```python
from build123d import *

# Parameters (mm, degrees)
SKETCH1_W            = 20
SKETCH1_H            = 40
BOSS_EXTRUDE1_DEPTH  = 5
SKETCH2_W            = 20
SKETCH2_H            = 20
BOSS_EXTRUDE2_DEPTH  = 20
SKETCH3_W            = 6
SKETCH3_H            = 16
CUT_EXTRUDE1_DEPTH   = 20
M3_CLEARANCE_HOLE1_D = 3.4
SKETCH6_W            = 20
SKETCH6_H            = 5
BOSS_EXTRUDE3_DEPTH  = 60
SKETCH7_W            = 20
SKETCH7_H            = 5
BOSS_EXTRUDE4_DEPTH  = 20
SKETCH8_W            = 20
SKETCH8_H            = 20
BOSS_EXTRUDE5_DEPTH  = 20
SKETCH9_W            = 6
SKETCH9_H            = 16
CUT_EXTRUDE2_DEPTH   = 20
M3_CLEARANCE_HOLE2_D = 3.4


with BuildPart() as part:
    # Sketch1 → Boss-Extrude1 (new body)
    with BuildSketch(Plane(origin=(0, 0, 0), x_dir=(1, 0, 0), z_dir=(0, 1, 0))):
        Rectangle(SKETCH1_W, SKETCH1_H)
    extrude(amount=BOSS_EXTRUDE1_DEPTH)

    # Sketch2 → Boss-Extrude2 (add)
    with BuildSketch(Plane(origin=(0, 0, 0), x_dir=(-1, 0, 0), z_dir=(0, -1, 0))):
        with Locations((0, 10)):
            Rectangle(SKETCH2_W, SKETCH2_H)
    extrude(amount=BOSS_EXTRUDE2_DEPTH)

    # Sketch3 → Cut-Extrude1 (cut)
    with BuildSketch(Plane(origin=(0, -20, 0), x_dir=(-1, 0, 0), z_dir=(0, -1, 0))):
        with Locations((0, 12)):
            Rectangle(SKETCH3_W, SKETCH3_H)
    extrude(amount=-CUT_EXTRUDE1_DEPTH, mode=Mode.SUBTRACT)

    # M3 Clearance Hole1 (through all)
    with Locations(Plane(origin=(0, 0, 0), x_dir=(-1, 0, 0), z_dir=(0, -1, 0))):
        with Locations((-5.5, -9.5), (5.5, -9.5)):
            Hole(M3_CLEARANCE_HOLE1_D / 2)

    # Sketch6 → Boss-Extrude3 (add)
    with BuildSketch(Plane(origin=(0, 0, -20), x_dir=(-1, 0, 0), z_dir=(0, 0, -1))):
        with Locations((0, 2.5)):
            Rectangle(SKETCH6_W, SKETCH6_H)
    extrude(amount=BOSS_EXTRUDE3_DEPTH)

    # Sketch7 → Boss-Extrude4 (add)
    with BuildSketch(Plane(origin=(0, 0, -80), x_dir=(-1, 0, 0), z_dir=(0, 0, -1))):
        with Locations((0, 2.5)):
            Rectangle(SKETCH7_W, SKETCH7_H)
    extrude(amount=BOSS_EXTRUDE4_DEPTH)

    # Sketch8 → Boss-Extrude5 (add)
    with BuildSketch(Plane(origin=(0, 0, 0), x_dir=(-1, 0, 0), z_dir=(0, -1, 0))):
        with Locations((0, 70)):
            Rectangle(SKETCH8_W, SKETCH8_H)
    extrude(amount=BOSS_EXTRUDE5_DEPTH)

    # Sketch9 → Cut-Extrude2 (cut)
    with BuildSketch(Plane(origin=(0, -20, 0), x_dir=(-1, 0, 0), z_dir=(0, -1, 0))):
        with Locations((0, 68)):
            Rectangle(SKETCH9_W, SKETCH9_H)
    extrude(amount=-CUT_EXTRUDE2_DEPTH, mode=Mode.SUBTRACT)

    # M3 Clearance Hole2 (through all)
    with Locations(Plane(origin=(0, 0, 0), x_dir=(-1, 0, 0), z_dir=(0, -1, 0))):
        with Locations((-5.5, 89.5), (5.5, 89.5)):
            Hole(M3_CLEARANCE_HOLE2_D / 2)


solid = part.part
```
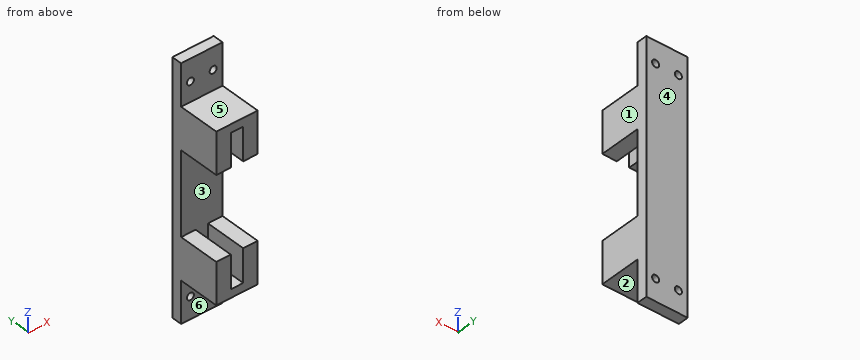
Source: CAD feature listing. Evaluate the final solid. Frame: model axes, mm. Face numbers are marked on the shaded views. A direction names the side the tool comes from. Round coordinates to 2 decimals unless told otherwise and drop trailing zeros. Loops run counter-clockwise (first coordinate to the right, second up) from the corner with the lowest first, then second, coordinate; pieces in that order, holes last.
1. Contact query for flat-ended pins moving along their axis: pin 1 (3.5 mm diameter, centred on x = 7.5, y = -8, fed in from +Z); pin 2 (3 mm diameter, centred on x = -5.5, z = -89.5, fed in from -Y); pin 3 (3.5 mm diameter, centred on x = 6.5, y = -6, fed in from -Z); pin 4 (4 mm diameter, centred on x = -5.5, z = 9.5, fed in from -Y). Output: stop coordinate, or through.
2. Mould query, pull axis X, two halves, no side actions, for the marked faces 1, 2 and 3. Classes: released by +X, released by -X, zero draft, split by the parting line, or undercut.
3. Section query A-A on y = -11.5. Output: boundary loops of the cut face in (x, z).
4. Section query B-B on z = -89.5. Output: boundary loops of the cut face in (x, y), and give its area (3 significant figures).
5. Ray query, L1, parallel to Z at x = -5.5, y = 3.5; L2, parallel to X at y = 1.2, z = 9.5; L3, parallel to Z at x = -5, y = -4.5. Return the intervals inside material, ascending.
6. Section query C-C on x = 5.5. Output: boundary loops of the cut face in (y, z).
7. Section query D-D on y = 2.5. Output: boundary loops of the cut face in (x, z), and give its area (3 significant figures).
8. Access query for the marked faces 4, 5 and 6. Directions: +Z, -Z, +X, -X, +Y, -Y. A direction counts if a zero-diameter tool reaches every point of the face in a straight line with its end or side. Return the directions, or none.
Answers below:
1. pin 1: stops at z = 0
1. pin 2: passes through
1. pin 3: stops at z = -80
1. pin 4: stops at y = 0
2. face 1: released by +X
2. face 2: zero draft
2. face 3: undercut
3. outline: (-10, -80) - (10, -80) - (10, -60) - (3, -60) - (3, -76) - (-3, -76) - (-3, -60) - (-10, -60) - close; (-10, -20) - (-3, -20) - (-3, -4) - (3, -4) - (3, -20) - (10, -20) - (10, 0) - (-10, 0) - close
4. outline: (-10, 0) - (-7.2, 0) - (-7.2, 5) - (-10, 5) - close; (-3.8, 0) - (3.8, 0) - (3.8, 5) - (-3.8, 5) - close; (7.2, 0) - (10, 0) - (10, 5) - (7.2, 5) - close
4. area: 66.0 mm2
5. L1: z = -100 to -91.2, -87.8 to 7.8, 11.2 to 20
5. L2: x = -10 to -7.2, -3.8 to 3.8, 7.2 to 10
5. L3: z = -80 to -60, -20 to 0
6. outline: (-20, -80) - (0, -80) - (0, -87.8) - (5, -87.8) - (5, 7.8) - (0, 7.8) - (0, 0) - (-20, 0) - (-20, -20) - (0, -20) - (0, -60) - (-20, -60) - close; (0, -100) - (5, -100) - (5, -91.2) - (0, -91.2) - close; (0, 11.2) - (5, 11.2) - (5, 20) - (0, 20) - close
7. outline: (-10, -100) - (10, -100) - (10, 20) - (-10, 20) - close; hole circle Ø3.4 at (-5.5, -89.5); hole circle Ø3.4 at (-5.5, 9.5); hole circle Ø3.4 at (5.5, -89.5); hole circle Ø3.4 at (5.5, 9.5)
7. area: 2,360 mm2
8. face 4: +Z, -Z, +X, -X, +Y
8. face 5: +Z, +X, -X, -Y
8. face 6: -Z, +X, -X, -Y
